Read the model definition and answer for the solid it produces. Units are mm, in the model's axes. Face numbers are marked on the shaded views. A direction names the side the tool comes from. Round coordinates to 2 decimals unless told otherwise and drop trailing zeros. Write each loop counter-clockwise with the first axis right and the second up, starting at its lowest first coordinate (ties: lowest second). Pieces come first, ordered by that corner, then holes. Notation, with made-up numbers: (-22.5, 55.5) - (34.5, 55.5) arc R23 ccw to (34.5, 86.5) - close; hole circle Ø11 at (2.5, 86.5). An arc over 180 degrees is marked (long way). Answer as CSV lines item,"result". Start each with the question number.
1) Consider line 1 along Z through (x, y) = (0, 12.75); line 2 along Z through (x, y) = (0, 8.75). Determine where each line is inside the solid, lowest interval first.
2) Which of the six approach directions +Z, -Z, +X, -X, +Y, -Y give full straight-line access (tool end or side, diameter ignored) to the marked faces 4, 5 and 6?
3) Find section A-A on x = 0. Determine the outline of the cut face in (y, z), then the cut area to 3 significant figures.
4) Each of these flat-tipped pins is pushed along its axis until it touches: pin 1 (4 mm diameter, centred on y = 21.5, z = 0.5, fed in from -X); pin 2 (3 mm diameter, centred on x = 7, y = 20.5, fed in from -Z); pin 3 (2 mm diameter, centred on x = 7.5, y = 19, fed in from -Z). Where does it stop, or does it pass through?
5) Find section D-D on x = -9.75. Determine the outline of the cut face in (y, z).
6) For a pull along X with two mould halves and no side action, classify the marked faces 1, 2 and 3 as +X half, -X half, draft (parallel to the pull), parting line (faces both ways), or undercut.
7) Find section B-B on z = 0. Determine the outline of the cut face in (x, y).
8) Find section C-C on y = 17.5. Determine the outline of the cut face in (x, z).
from build123d import *

# Parameters (mm, degrees)
SKETCH1_R           = 14
BOSS_EXTRUDE1_DEPTH = 1.5
SKETCH2_R           = 11.85
BOSS_EXTRUDE2_DEPTH = 11
SKETCH3_R           = 14
BOSS_EXTRUDE3_DEPTH = 1.5
SKETCH4_R           = 8.5
BOSS_EXTRUDE4_DEPTH = 11
SKETCH5_R           = 4
CUT_EXTRUDE1_DEPTH  = 26


with BuildPart() as part:
    # Sketch1 → Boss-Extrude1 (new body)
    with BuildSketch(Plane(origin=(0, 0, 0), x_dir=(1, 0, 0), z_dir=(0, 1, 0))):
        Circle(SKETCH1_R)
    extrude(amount=BOSS_EXTRUDE1_DEPTH)

    # Sketch2 → Boss-Extrude2 (add)
    with BuildSketch(Plane(origin=(0, 1.5, 0), x_dir=(1, 0, 0), z_dir=(0, 1, 0))):
        Circle(SKETCH2_R)
    extrude(amount=BOSS_EXTRUDE2_DEPTH)

    # Sketch3 → Boss-Extrude3 (add)
    with BuildSketch(Plane(origin=(0, 12.5, 0), x_dir=(1, 0, 0), z_dir=(0, 1, 0))):
        Circle(SKETCH3_R)
    extrude(amount=BOSS_EXTRUDE3_DEPTH)

    # Sketch4 → Boss-Extrude4 (add)
    with BuildSketch(Plane(origin=(0, 14, 0), x_dir=(1, 0, 0), z_dir=(0, 1, 0))):
        Circle(SKETCH4_R)
    extrude(amount=BOSS_EXTRUDE4_DEPTH)

    # Sketch5 → Cut-Extrude1 (cut, through all)
    with BuildSketch(Plane(origin=(0, 25, 0), x_dir=(1, 0, 0), z_dir=(0, 1, 0))):
        Circle(SKETCH5_R)
    extrude(amount=-CUT_EXTRUDE1_DEPTH, mode=Mode.SUBTRACT)


solid = part.part
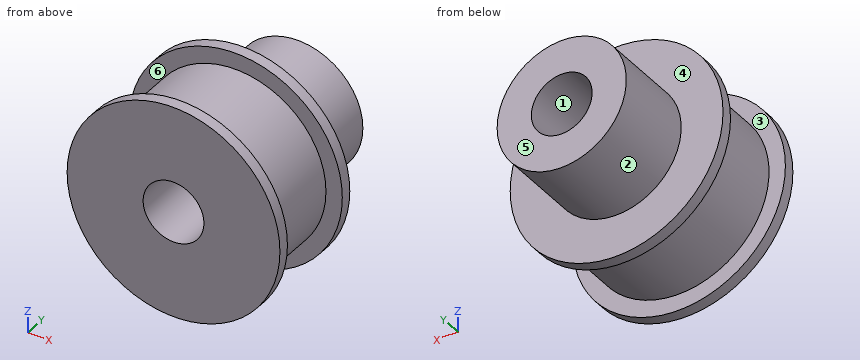
Check values:
1,line 1,"z = -14 to -4, 4 to 14"
1,line 2,"z = -11.85 to -4, 4 to 11.85"
2,face 4,"+Y"
2,face 5,"+Z, -Z, +X, -X, +Y"
2,face 6,"none"
3,outline,"(0, -14) - (1.5, -14) - (1.5, -11.85) - (12.5, -11.85) - (12.5, -14) - (14, -14) - (14, -8.5) - (25, -8.5) - (25, -4) - (0, -4) - close; (0, 4) - (25, 4) - (25, 8.5) - (14, 8.5) - (14, 14) - (12.5, 14) - (12.5, 11.85) - (1.5, 11.85) - (1.5, 14) - (0, 14) - close"
3,area,"332 mm^2"
4,pin 1,"stops at x = -8.5"
4,pin 2,"stops at z = -6.48"
4,pin 3,"stops at z = -5.48"
5,outline,"(0, -10.05) - (1.5, -10.05) - (1.5, -6.73) - (12.5, -6.73) - (12.5, -10.05) - (14, -10.05) - (14, 10.05) - (12.5, 10.05) - (12.5, 6.73) - (1.5, 6.73) - (1.5, 10.05) - (0, 10.05) - close"
6,face 1,"undercut"
6,face 2,"parting line"
6,face 3,"draft"
7,outline,"(-14, 0) - (-4, 0) - (-4, 25) - (-8.5, 25) - (-8.5, 14) - (-14, 14) - (-14, 12.5) - (-11.85, 12.5) - (-11.85, 1.5) - (-14, 1.5) - close; (4, 0) - (14, 0) - (14, 1.5) - (11.85, 1.5) - (11.85, 12.5) - (14, 12.5) - (14, 14) - (8.5, 14) - (8.5, 25) - (4, 25) - close"
8,outline,"circle Ø17 at (0, 0); hole circle Ø8 at (0, 0)"
